Source: CAD feature listing. Evaluate the final solid. Frame: model axes, mm. A direction names the side the tool comes from. Round coordinates to 2 decimals unless told otherwise and drop trailing zeros. Order: outer loops, then holes, each group sorted by start corner. A loop starts at its lowest first (then second) coordinate and runs counter-clockwise, first axis right, second up. Notation, with made-up numbers: M 41.5,-32 L 72.5,-32 A23 cw 72.5,-19 Z; hole C 4.25,36.25 d3. An arc over 180 degrees is marked long. Answer in a Markdown table with one row per item. Add a question column.
Autodesk Fusion 360 part; units mm, degrees
sketch "Sketch1" plane through (0, 0, 0) normal (0, 0, 1) x (1, 0, 0)
  line L0 (-39.3784, 42.4452) -> (-27.3784, 42.4452)
  line L1 (-27.3784, 42.4452) -> (-27.3784, 15.4452)
  line L2 (-27.3784, 15.4452) -> (-39.3784, 15.4452)
  line L3 (-39.3784, 15.4452) -> (-39.3784, 42.4452)
  dimension "d1" = 12
  dimension "d2" = 27
extrude "Extrude1" add sketch "Sketch1" along normal blind 3
sketch "Sketch2" plane through (0, 0, 3) normal (0, 0, 1) x (-1, 0, 0)
  line L0 (39.3784, -15.4452) -> (27.3784, -15.4452)
  line L1 (27.3784, -15.4452) -> (27.3784, -42.4452)
  line L2 (27.3784, -42.4452) -> (39.3784, -42.4452)
  line L3 (39.3784, -42.4452) -> (39.3784, -15.4452)
  circle A0 centre (33.3784, -28.9452) radius 4.25
  dimension "d5" = 8.5
extrude "Extrude2" add sketch "Sketch2" along normal blind 4.5 contours A0
sketch "Sketch3" plane through (0, 0, 0) normal (0, 0, -1) x (1, 0, 0)
  line L0 (-27.3784, -15.4452) -> (-39.3784, -15.4452)
  line L1 (-39.3784, -15.4452) -> (-39.3784, -42.4452)
  line L2 (-39.3784, -42.4452) -> (-27.3784, -42.4452)
  line L3 (-27.3784, -42.4452) -> (-27.3784, -15.4452)
  line L4 (-33.3784, -15.4452) -> (-30.8784, -15.4452) construction
  line L5 (-30.8784, -15.4452) -> (-35.8784, -15.4452)
  line L6 (-35.8784, -15.4452) -> (-35.8784, -42.4452)
  line L7 (-35.8784, -42.4452) -> (-30.8784, -42.4452)
  line L8 (-30.8784, -42.4452) -> (-30.8784, -15.4452)
  line L9 (-30.8784, -28.9452) -> (-30.8784, -24.9452) construction
  line L10 (-30.8784, -24.9452) -> (-35.8784, -24.9452)
  line L11 (-35.8784, -24.9452) -> (-35.8784, -32.9452)
  line L12 (-35.8784, -32.9452) -> (-30.8784, -32.9452)
  line L13 (-30.8784, -32.9452) -> (-30.8784, -24.9452)
  circle A0 centre (-33.3784, -32.9452) radius 2.5
  circle A1 centre (-33.3784, -24.9452) radius 2.5
  dimension "d8" = 2.5
  dimension "d9" = 5
  dimension "d10" = 4
  dimension "d11" = 8
extrude "Extrude3" cut sketch "Sketch3" against normal blind 15 contours L10 A1 | L10 A1 | L6 L8 L11 L13 A0 A1 | L12 A0 | L12 A0
sketch "Sketch4" plane through (-35.8784, 0, 0) normal (1, 0, 0) x (0, 1, 0)
  line L0 (25.5083, 3) -> (24.9452, 3)
  line L1 (24.9452, 3) -> (24.9452, 0)
  line L2 (24.9452, 0) -> (32.9452, 0)
  line L3 (32.9452, 0) -> (32.9452, 3)
  line L4 (32.9452, 3) -> (32.3821, 3)
  line L5 (32.3821, 3) -> (32.3821, 7.5)
  line L6 (32.3821, 7.5) -> (25.5083, 7.5)
  line L7 (25.5083, 7.5) -> (25.5083, 3)
sketch "Sketch5" plane through (0, 0, 0) normal (0, 0, -1) x (1, 0, 0)
  line L0 (-35.8784, -32.9452) -> (-35.8784, -24.9452)
  arc A0 (-30.8784, -24.9452) -> (-35.8784, -24.9452) centre (-33.3784, -24.9452) ccw
  line L1 (-30.8784, -24.9452) -> (-30.8784, -32.9452)
  arc A1 (-35.8784, -32.9452) -> (-30.8784, -32.9452) centre (-33.3784, -32.9452) ccw
  line L2 (-27.3784, -15.4452) -> (-39.3784, -15.4452)
  line L3 (-39.3784, -15.4452) -> (-39.3784, -42.4452)
  line L4 (-39.3784, -42.4452) -> (-27.3784, -42.4452)
  line L5 (-27.3784, -42.4452) -> (-27.3784, -15.4452)
  line L6 (-39.3784, -42.4452) -> (-27.3784, -42.4452)
  line L7 (-27.3784, -42.4452) -> (-27.3784, -38.4452)
  line L8 (-27.3784, -38.4452) -> (-39.3784, -38.4452)
  line L9 (-39.3784, -38.4452) -> (-39.3784, -42.4452)
  line L10 (-39.3784, -15.4452) -> (-27.3784, -15.4452)
  line L11 (-27.3784, -15.4452) -> (-27.3784, -19.4452)
  line L12 (-27.3784, -19.4452) -> (-39.3784, -19.4452)
  line L13 (-39.3784, -19.4452) -> (-39.3784, -15.4452)
  dimension "d14" = 4
  dimension "d15" = 4
extrude "Extrude4" add sketch "Sketch5" along normal blind 25 contours L2 L3 L5 L10 L11 L12 L13 | L3 L4 L5 L6 L7 L8 L9
sketch "Sketch6" plane through (-27.3784, 0, 0) normal (1, 0, 0) x (0, 1, 0)
  line L0 (42.4452, -25) -> (42.4452, 3)
  line L1 (42.4452, 3) -> (15.4452, 3)
  line L2 (15.4452, 3) -> (15.4452, -25)
  line L3 (15.4452, -25) -> (19.4452, -25)
  line L4 (19.4452, -25) -> (19.4452, 0)
  line L5 (19.4452, 0) -> (38.4452, 0)
  line L6 (38.4452, 0) -> (38.4452, -25)
  line L7 (38.4452, -25) -> (42.4452, -25)
  line L8 (19.4452, 0) -> (15.4452, 0)
  line L9 (38.4452, 0) -> (42.4452, 0)
extrude "Extrude5" add sketch "Sketch6" along normal blind 4 contours L0 L6 L7 L9 | L2 L3 L4 L8
sketch "Sketch7" plane through (-39.3784, 0, 0) normal (-1, 0, 0) x (0, -1, 0)
  line L0 (-15.4452, -25) -> (-15.4452, 3)
  line L1 (-15.4452, 3) -> (-42.4452, 3)
  line L2 (-42.4452, 3) -> (-42.4452, -25)
  line L3 (-42.4452, -25) -> (-38.4452, -25)
  line L4 (-38.4452, -25) -> (-38.4452, 0)
  line L5 (-38.4452, 0) -> (-19.4452, 0)
  line L6 (-19.4452, 0) -> (-19.4452, -25)
  line L7 (-19.4452, -25) -> (-15.4452, -25)
  line L8 (-42.4452, 0) -> (-15.4452, 0)
extrude "Extrude6" add sketch "Sketch7" along normal blind 4 contours L0 L6 L7 L8 | L2 L3 L4 L8
sketch "Sketch8" plane through (0, 15.4452, 0) normal (0, -1, 0) x (1, 0, 0)
  line L0 (-27.3784, 0) -> (-27.3784, 3)
  line L1 (-27.3784, 3) -> (-39.3784, 3)
  line L2 (-39.3784, 3) -> (-39.3784, 0)
  line L3 (-39.3784, 0) -> (-43.3784, 0)
  line L4 (-43.3784, 0) -> (-43.3784, -25)
  line L5 (-43.3784, -25) -> (-23.3784, -25)
  line L6 (-23.3784, -25) -> (-23.3784, 0)
  line L7 (-23.3784, 0) -> (-27.3784, 0)
  line L8 (-39.3784, 0) -> (-27.3784, 0)
extrude "Extrude7" add sketch "Sketch8" along normal blind 11 contours L3 L4 L5 L6 L7 L8
sketch "Sketch9" plane through (0, 42.4452, 0) normal (0, 1, 0) x (-1, 0, 0)
  line L0 (39.3784, 0) -> (39.3784, 3)
  line L1 (39.3784, 3) -> (27.3784, 3)
  line L2 (27.3784, 3) -> (27.3784, 0)
  line L3 (27.3784, 0) -> (23.3784, 0)
  line L4 (23.3784, 0) -> (23.3784, -25)
  line L5 (23.3784, -25) -> (43.3784, -25)
  line L6 (43.3784, -25) -> (43.3784, 0)
  line L7 (43.3784, 0) -> (39.3784, 0)
  line L8 (27.3784, 0) -> (39.3784, 0)
extrude "Extrude8" add sketch "Sketch9" along normal blind 11 contours L3 L4 L5 L6 L7 L8
sketch "Sketch10" plane through (0, 53.4452, 0) normal (0, 1, 0) x (-1, 0, 0)
  line L0 (23.3784, 0) -> (23.3784, -25)
  line L1 (23.3784, -25) -> (43.3784, -25)
  line L2 (43.3784, -25) -> (43.3784, 0)
  line L3 (43.3784, 0) -> (23.3784, 0)
  line L4 (33.3784, 0) -> (33.3784, -10.5) construction
  circle A0 centre (33.3784, -10.5) radius 10
  dimension "d26" = 10.5
  dimension "d27" = 20
extrude "Extrude9" cut sketch "Sketch10" against normal blind 62 contours A0
extrude "Extrude10" add 4 faces at (-23.3784, 48.4452, -3.5) (-23.3784, 9.4452, -7) (-23.3784, 14.4452, -20.1667) (-23.3784, 48.4452, -20.1667) along direction (1, 0, 0) blind 0.5
extrude "Extrude11" add 4 faces at (-43.3784, 43.4452, -3.5) (-43.3784, 48.4452, -20.1667) (-43.3784, 14.4452, -15.3333) (-43.3784, 14.4452, -3.5) along direction (-1, 0, 0) blind 0.5
extrude "Extrude12" add 1 faces at (-33.1293, 38.4452, -23.4907) along direction (0, -1, 0) blind 1
extrude "Extrude13" add 1 faces at (-33.1293, 19.4452, -23.4907) along direction (0, 1, 0) blind 1
extrude "Extrude14" add 1 faces at (-43.8784, 42.7785, -8.3333) along direction (-1, 0, 0) blind 2
extrude "Extrude15" add 1 faces at (-43.8784, 15.1119, -8.3333) along direction (-1, 0, 0) blind 2
extrude "Extrude16" add 1 faces at (-22.8784, 42.7785, -16.6667) along direction (1, 0, 0) blind 2
extrude "Extrude17" add 1 faces at (-22.8784, 15.1119, -8.3333) along direction (1, 0, 0) blind 2
extrude "Extrude18" cut 1 faces at (-33.1293, 4.4452, -23.4907) along direction (0, 1, 0) blind 1
extrude "Extrude19" cut 1 faces at (-33.1293, 53.4452, -23.4907) along direction (0, -1, 0) blind 1
extrude "Extrude20" add 2 faces at (-30.1717, 28.772, 7.5) (-36.576, 27.9712, 7.5) along direction (0, 0, 1) blind 0.5
sketch "Sketch11" plane through (0, 52.4452, 0) normal (0, 1, 0) x (-1, 0, 0)
  line L0 (45.8784, 0) -> (20.8784, 0)
  line L1 (20.8784, 0) -> (20.8784, -25)
  line L2 (20.8784, -25) -> (45.8784, -25)
  line L3 (45.8784, -25) -> (45.8784, 0)
  circle A0 centre (33.3784, -10.5) radius 10
  line L4 (45.8784, 0) -> (44.1284, 0)
  line L5 (44.1284, 0) -> (44.1284, -25)
  line L6 (44.1284, -25) -> (45.8784, -25)
  line L7 (45.8784, -25) -> (45.8784, 0)
  dimension "d52" = 1.75
extrude "Extrude21" add sketch "Sketch11" against normal blind 47 contours L0 L2 L3 L4 L5 L6 L7
extrude "Extrude22" cut 2 faces at (-20.8784, 47.4452, -16.6667) (-20.8784, 10.4452, -8.3333) along direction (-1, 0, 0) blind 1
sketch "Sketch12" plane through (0, 52.4452, 0) normal (0, 1, 0) x (-1, 0, 0)
  line L0 (21.8784, 0) -> (21.8784, -25)
  line L1 (21.8784, -25) -> (45.8784, -25)
  line L2 (45.8784, -25) -> (45.8784, 0)
  line L3 (45.8784, 0) -> (21.8784, 0)
  circle A0 centre (33.3784, -10.5) radius 10
  circle A1 centre (33.3784, -10.5) radius 10.125
  dimension "d67" = 20.25
extrude "Extrude25" cut sketch "Sketch12" against normal blind 68 contours A1
sketch "Sketch13" plane through (0, 0, -25) normal (0, 0, -1) x (1, 0, 0)
  line L0 (-21.8784, -52.4452) -> (-21.8784, -37.4452)
  line L1 (-21.8784, -37.4452) -> (-44.1284, -37.4452)
  line L2 (-44.1284, -37.4452) -> (-44.1284, -20.4452)
  line L3 (-44.1284, -20.4452) -> (-21.8784, -20.4452)
  line L4 (-21.8784, -20.4452) -> (-21.8784, -5.4452)
  line L5 (-21.8784, -5.4452) -> (-45.8784, -5.4452)
  line L6 (-45.8784, -5.4452) -> (-45.8784, -52.4452)
  line L7 (-45.8784, -52.4452) -> (-21.8784, -52.4452)
  line L8 (-45.8784, -52.4452) -> (-33.3784, -52.4452) construction
  line L9 (-33.3784, -52.4452) -> (-35.3784, -52.4452) construction
  line L10 (-35.3784, -52.4452) -> (-31.3784, -52.4452)
  line L11 (-31.3784, -52.4452) -> (-31.3784, -48.4452)
  line L12 (-31.3784, -48.4452) -> (-35.3784, -48.4452)
  line L13 (-35.3784, -48.4452) -> (-35.3784, -52.4452)
  dimension "d57" = 12.5
  dimension "d58" = 2
  dimension "d59" = 4
  dimension "d60" = 4
extrude "Extrude23" cut sketch "Sketch13" against normal blind 10 contours L7 L10 L11 L12 L13
sketch "Sketch14" plane through (0, 0, -25) normal (0, 0, -1) x (1, 0, 0)
  line L0 (-35.3784, -52.4452) -> (-35.3784, -48.4452)
  line L1 (-35.3784, -48.4452) -> (-31.3784, -48.4452)
  line L2 (-31.3784, -48.4452) -> (-31.3784, -52.4452)
  line L3 (-31.3784, -52.4452) -> (-21.8784, -52.4452)
  line L4 (-21.8784, -52.4452) -> (-21.8784, -37.4452)
  line L5 (-21.8784, -37.4452) -> (-44.1284, -37.4452)
  line L6 (-44.1284, -37.4452) -> (-44.1284, -20.4452)
  line L7 (-44.1284, -20.4452) -> (-21.8784, -20.4452)
  line L8 (-21.8784, -20.4452) -> (-21.8784, -5.4452)
  line L9 (-21.8784, -5.4452) -> (-45.8784, -5.4452)
  line L10 (-45.8784, -5.4452) -> (-45.8784, -52.4452)
  line L11 (-45.8784, -52.4452) -> (-35.3784, -52.4452)
  line L12 (-35.3784, -48.4452) -> (-35.3784, -5.4452) construction
  line L13 (-35.3784, -5.4452) -> (-31.3784, -5.4452)
  line L14 (-31.3784, -5.4452) -> (-31.3784, -9.4452)
  line L15 (-31.3784, -9.4452) -> (-35.3784, -9.4452)
  line L16 (-35.3784, -9.4452) -> (-35.3784, -5.4452)
  dimension "d63" = 4
  dimension "d64" = 4
extrude "Extrude24" cut sketch "Sketch14" against normal blind 7 contours L9 L13 L14 L15 L16
(1) Draft query along Y for faces 6 (the face through (-33.433, 35.445, 1.479)), 7 (the face through (-45, 29, 0)), 8 (the face through (-37.63, 28.89, 5.46)). Return one class per face: +Y half, -Y half, draft (parallel to the pull), parting line (faces both ways), or undercut.
(2) Cut plane A-A (z = 2.5). Return loops of the section in (x, y), and give its area (3 significant figures).
(3) Cut plane B-B (x = -26.75). Return loops of the section in (y, z), and give its area (3 significant figures).
(4) Line query: line 1 (X direction, y = 42.5, z = -10.5); line 2 (Y direction, x = -43.75, z = -22.5); line 3 (X direction, y = 26, z = -6.5). Output: solid intervals per line, ascending. Write a range as from..to.
(5) Cut plane D-D (y = 14). Return loops of the section in (x, z) (3 decimals).
(6) Cut plane C-C (z = -6). Return loops of the section in (x, y).
(7) Pin query (flat end, axial travel): pin 1 (1.5 mm diameter, centred on y = 25.5, z = 1.5, fed in from +X); pin 2 (10 mm diameter, centred on x = -34, y = 28, fed in from -Z); pin 3 (6.5 mm diameter, centred on y = 27.5, z = 4.5, fed in from -X). Return the tip coordinate at first contact, or that it passes through.
(8) Access query for faces 1 (the face through (-33, 42.445, 1)), 2 (the face through (-27.378, 29, 1)), 3 (the face through (-33.323, 22.446, 1.479)), 4 (the face through (-39.378, 29, 1)), 5 (the face through (-33, 37.445, -21)). Directions: +Z, -Z, +X, -X, +Y, -Y. A direction counts if a zero-diameter tool reaches every point of the face in a straight line with its end or side. Return the directions, or none.
Answer list:
| question | item | result |
|---|---|---|
| 1 | face 6 | undercut |
| 1 | face 7 | draft |
| 1 | face 8 | parting line |
| 2 | outline | M -39.38,15.45 L -27.38,15.45 L -27.38,42.45 L -39.38,42.45 Z; hole M -35.88,24.95 A2.5 ccw -30.88,24.95 L -30.88,32.95 A2.5 ccw -35.88,32.95 Z |
| 2 | area | 264 mm² |
| 3 | outline | M 5.45,-25 L 20.45,-25 L 20.45,-18.15 L 5.45,-18.15 Z; M 5.45,-2.85 L 20.45,-2.85 L 20.45,0 L 5.45,0 Z; M 37.45,-25 L 52.45,-25 L 52.45,-18.15 L 37.45,-18.15 Z; M 37.45,-2.85 L 52.45,-2.85 L 52.45,0 L 37.45,0 Z |
| 3 | area | 291 mm² |
| 4 | line 1 | -45.88..-43.5, -23.25..-21.88 |
| 4 | line 2 | 5.45..20.45, 37.45..52.45 |
| 4 | line 3 | -45.88..-44.13 |
| 5 | outline | M -45.878,-25 L -21.878,-25 L -21.878,0 L -45.878,0 Z; hole C -33.378,-10.5 d20.25 |
| 6 | outline | M -45.88,5.45 L -42.45,5.45 L -42.45,20.45 L -44.13,20.45 L -44.13,37.45 L -42.45,37.45 L -42.45,52.45 L -45.88,52.45 Z; M -24.31,5.45 L -21.88,5.45 L -21.88,20.45 L -24.31,20.45 Z; M -24.31,37.45 L -21.88,37.45 L -21.88,52.45 L -24.31,52.45 Z |
| 7 | pin 1 | x = -27.38 |
| 7 | pin 2 | z = 0 |
| 7 | pin 3 | x = -39.38 |
| 8 | face 1 | +Z, +X, -X, +Y |
| 8 | face 2 | +Z, +X, +Y, -Y |
| 8 | face 3 | +Z, -Z |
| 8 | face 4 | +Z, -X, +Y, -Y |
| 8 | face 5 | -Z, +X |
